from build123d import *

# Parameters (mm, degrees)
SKETCH1_W           = 300.2
SKETCH1_H           = 20
BOSS_EXTRUDE1_DEPTH = 20
FILLET1_R           = 2
SKETCH2_W           = 16
SKETCH2_H           = 16
CUT_EXTRUDE1_DEPTH  = 301.2


with BuildPart() as part:
    # Sketch1 → Boss-Extrude1 (new body)
    with BuildSketch(Plane.XY):
        with Locations((-440, -302)):
            Rectangle(SKETCH1_W, SKETCH1_H)
    extrude(amount=-BOSS_EXTRUDE1_DEPTH)

    # Fillet1
    fillet1_edges = [part.edges().sort_by_distance(p)[0] for p in [
        (-440, -312, -20),
        (-440, -312, 0),
        (-440, -292, 0),
        (-440, -292, -20),
    ]]
    fillet(fillet1_edges, radius=FILLET1_R)

    # Sketch2 → Cut-Extrude1 (cut, through all)
    with BuildSketch(Plane(origin=(-289.9, 0, 0), x_dir=(0, 0, -1), z_dir=(1, 0, 0))):
        with Locations((10, -302)):
            Rectangle(SKETCH2_W, SKETCH2_H)
    extrude(amount=-CUT_EXTRUDE1_DEPTH, mode=Mode.SUBTRACT)


solid = part.part
Model file for the job. Use its own axes, mm. A direction names the side the tool comes from. Give positions to 0.01 mm unless a question says otherwise; leave off trailing zeros. Loops run counter-clockwise (first coordinate to the right, second up) from the corner with the lowest first, then second, coordinate; pieces in that order, holes last.
1) Saw through at C-C (x = -394.5). Write the cut outline in (y, z), plus the area to 3 significant figures.
2) Saw through at A-A (z = -14). Write the cut outline in (x, y), plus the area to 3 significant figures.
3) Tool access for faces 1 (the flat face through (-590.1, -293, -10)), 2 (the flat face through (-438, -302, -2)): list every direction of +Z, -Z, +X, -X, +Y, -Y with a clear straight run to the whole face (end or side of a thin tool).
4) Wall check: line 1 (Z direction, x = -571, y = -304.5); line 2 (Y direction, x = -530, z = -9); line 3 (Y direction, x = -573.5, z = -1). Give the ranges that are in metal, low to high.
5) Saw through at B-B (y = -306). Write the cut outline in (x, z), plus the area to 3 significant figures.
6) Pull direction Z, two halves, no side cores. Call faces 3 (the flat face through (-438, -294, -10)), 4 (the flat face through (-289.9, -293, -10)), 5 (the flat face through (-442, -302, 0)): +Z half, -Z half, draft (parallel to the pull), parting line (faces both ways), or undercut.
Answer block:
1. outline: (-312, -18) arc R2 ccw to (-310, -20) - (-294, -20) arc R2 ccw to (-292, -18) - (-292, -2) arc R2 ccw to (-294, 0) - (-310, 0) arc R2 ccw to (-312, -2) - close; hole (-310, -18) - (-294, -18) - (-294, -2) - (-310, -2) - close
1. area: 141 mm2
2. outline: (-590.1, -312) - (-289.9, -312) - (-289.9, -310) - (-590.1, -310) - close; (-590.1, -294) - (-289.9, -294) - (-289.9, -292) - (-590.1, -292) - close
2. area: 1,200 mm2
3. face 1: +Z, -Z, -X, +Y, -Y
3. face 2: +X, -X
4. line 1: z = -20 to -18, -2 to 0
4. line 2: y = -312 to -310, -294 to -292
4. line 3: y = -311.73 to -292.27
5. outline: (-590.1, -20) - (-289.9, -20) - (-289.9, -18) - (-590.1, -18) - close; (-590.1, -2) - (-289.9, -2) - (-289.9, 0) - (-590.1, 0) - close
5. area: 1,200 mm2
6. face 3: undercut
6. face 4: draft
6. face 5: +Z half
